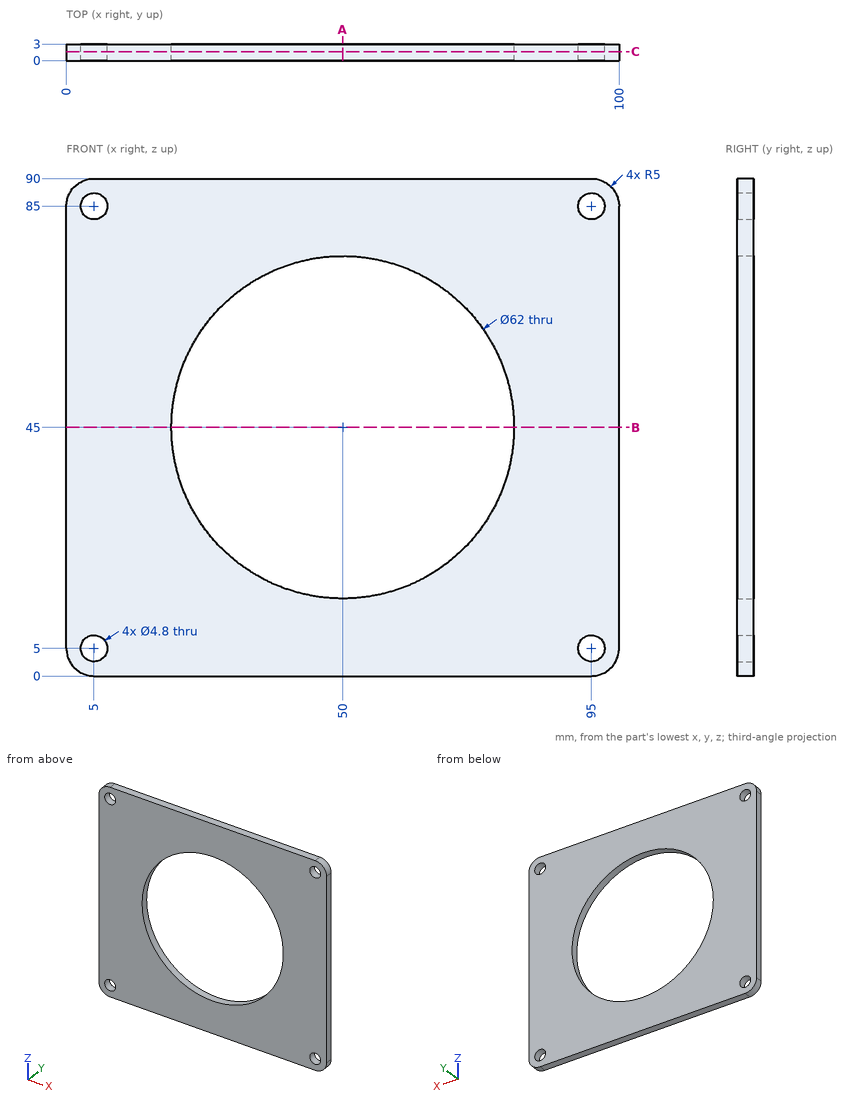
The drawing under review shows one solid part. Ordinate dimensions are in mm from its lowest x, y, z. Coordinates: 2 decimals unless noted, no trailing zeros. Order: outer loops, then holes, each group sorted by start corner. A loop starts at its lowest first (then second) coordinate and runs counter-clockwise, first axis right, second up. Notation, with made-up numbers: (36, 15) -> (57, 15) arc R35 cw to (57, 53) -> close; hole circle Ø11 at (-35, -3.5). An arc over 180 degrees is marked (long way). Answer in a Markdown table with one row per item.
(1) Insertion check: pin 1 (8 mm diameter, centred on x = 73, z = 62, fed in from -Y); pin 2 (4 mm diameter, centred on x = 5, z = 5, fed in from -Y). Each pin has a flat end and moves straight along its axis. Give the tip position at first contact, or say it passes through.
Answers:
| item | result |
|---|---|
| pin 1 | y = 0 |
| pin 2 | through |
(2) Consider section C-C (y = 1.6). Write out the cut boundary in (x, z), plus the area to 3 significant figures.
Answers:
| item | result |
|---|---|
| outline | (0, 5) arc R5 ccw to (5, 0) -> (95, 0) arc R5 ccw to (100, 5) -> (100, 85) arc R5 ccw to (95, 90) -> (5, 90) arc R5 ccw to (0, 85) -> close; hole circle Ø4.8 at (5, 5); hole circle Ø4.8 at (5, 85); hole circle Ø62 at (50, 45); hole circle Ø4.8 at (95, 5); hole circle Ø4.8 at (95, 85) |
| area | 5,890 mm² |
(3) Consider section A-A (x = 50). Write out the cut boundary in (y, z).
Answers:
| item | result |
|---|---|
| outline | (0, 0) -> (3, 0) -> (3, 14) -> (0, 14) -> close; (0, 76) -> (3, 76) -> (3, 90) -> (0, 90) -> close |
(4) Consider section B-B (z = 45). Write out the cut boundary in (x, y).
Answers:
| item | result |
|---|---|
| outline | (0, 0) -> (19, 0) -> (19, 3) -> (0, 3) -> close; (81, 0) -> (100, 0) -> (100, 3) -> (81, 3) -> close |
(5) Wall thickness on line 1 along Z through (x, y) = (95, 0.65); line 2 along Z through (x, y) = (50, 1.2); line 3 along X through (y, z) = (2.7, 84.5): over which ranges is each line inside the solid? List them lowest first.
Answers:
| item | result |
|---|---|
| line 1 | 0 to 2.6, 7.4 to 82.6, 87.4 to 90 |
| line 2 | 0 to 14, 76 to 90 |
| line 3 | 0 to 2.65, 7.35 to 92.65, 97.35 to 100 |
